from build123d import *


with BuildPart() as part:
    # Sweep1: sweep along a path in Sketch2
    with BuildLine(Plane(origin=(0, 0, 0), x_dir=(1, 0, 0), z_dir=(0, 1, 0))) as sweep1_path:
        Line((0, 0), (0, 14))
        ThreePointArc((0, 14), (-0.878679656, 16.121320344), (-3, 17))
        Line((-3, 17), (-47, 17))
    # Sketch1 → Sweep1 (sweep)
    with BuildSketch(Plane.XY):
        Polygon((0, 1.154700538), (-1, 0.577350269), (-1, -0.577350269), (0, -1.154700538), (1, -0.577350269), (1, 0.577350269), align=None)
    sweep(path=sweep1_path.line)


solid = part.part
Part model, mm, in its own coordinate system. A direction names the side the tool comes from. Round coordinates to 2 decimals unless told otherwise and drop trailing zeros. Write each loop counter-clockwise with the first axis right and the second up, starting at its lowest first coordinate (ties: lowest second). Pieces come first, ordered by that corner, then holes. Notation, with made-up numbers: (-9.5, 61.25) - (10.5, 61.25) arc R32 cw to (10.5, 91.25) - close; hole circle Ø8 at (12.5, 33.5). An arc over 180 degrees is marked (long way). Use CSV: the item, a comma, the result in double quotes.
Item 1: Flat gauge pins, fed straight in: P1, Ø6, axis at x = -14, z = -13.5, coming from the +Y side; P2, Ø0.9, axis at x = -25, y = 0, coming from the +Z side; P3, Ø0.9, axis at y = 0, z = -6.5, coming from the -X side; P4, Ø1, axis at x = -11.5, z = -15, coming from the +Y side. Where does each tip first touch, or does it go through?
Results list:
P1,"stops at y = 0.87"
P2,"stops at z = -16"
P3,"stops at x = -1"
P4,"passes through"
Item 2: Tool access for faces 1 (the flat face through (0.51, 0.86, -7.1)), 2 (the flat face through (-0.51, -0.86, -7.1)), 3 (the flat face through (-0.49, 0.87, -7.1)), 4 (the flat face through (-25, 0, -16)): list every direction of +Z, -Z, +X, -X, +Y, -Y with a clear straight run to the whole face (end or side of a thin tool).
Results list:
face 1,"+Z, -Z, +X, +Y"
face 2,"+Z, -X, -Y"
face 3,"+Z, -X, +Y"
face 4,"+Z, -X, +Y, -Y"
Item 3: Slice it at C-C, the plane x = -11.5. Write the cut outline in (y, z), then the cut area to 3 significant figures.
Results list:
outline,"(-1.15, -17) - (-0.58, -18) - (0.58, -18) - (1.15, -17) - (0.58, -16) - (-0.58, -16) - close"
area,"3.46 mm²"
Item 4: Wall check: L1, parallel to X at y = -0.5, z = -2.25; L2, parallel to Z at x = -12, y = 0.4; L3, parallel to X at y = -0.8, z = -12.25. Give the ranges that are in metal, low to high.
Results list:
L1,"x = -1 to 1"
L2,"z = -18 to -16"
L3,"x = -0.61 to 0.61"
Item 5: Slice it at A-A, the plane y = 0. Write the cut outline in (x, z), then the cut area to 3 significant figures.
Results list:
outline,"(-47, -18) - (-3, -18) arc R4 ccw to (1, -14) - (1, 0) - (-1, 0) - (-1, -14) arc R2 cw to (-3, -16) - (-47, -16) - close"
area,"125 mm²"
Item 6: Slice it at B-B, the plane z = -2.5. Write the cut outline in (x, y).
Results list:
outline,"(-1, -0.58) - (0, -1.15) - (1, -0.58) - (1, 0.58) - (0, 1.15) - (-1, 0.58) - close"
